```python
from build123d import *

# Parameters (mm, degrees)
ESBO_O7_R                = 1.65
RESSALTO_EXTRUS_O5_DEPTH = 8
RESSALTO_EXTRUS_O6_START = -8
ESBO_O10_R               = 1.65
RESSALTO_EXTRUS_O6_DEPTH = 8
ESBO_O8_R                = 5.5
CORTE_EXTRUS_O4_DEPTH    = 8
FILETE1_R                = 10
ESBO_O11_R               = 2.75
CORTE_EXTRUS_O5_DEPTH    = 3.5
ESBO_O14_R               = 1.75
CORTE_EXTRUS_O9_DEPTH    = 8
CORTE_EXTRUS_O10_DEPTH   = 4.9


with BuildPart() as part:
    # Esboço7 → Ressalto-extrusão5 (new body)
    with BuildSketch(Plane.XY):
        Polygon((-45.692156379, 16.70804449), (-45.692156379, -36.79195551), (6.807843621, -36.79195551), (6.807843621, 4.155908866), (3.801241904, 7.162510584), (3.84677581, 7.20804449), (3.807843621, 7.20804449), (3.807843621, 44.20804449), (-1.192156379, 49.20804449), (-23.192156379, 49.20804449), (-23.192156379, 16.70804449), align=None)
        with Locations((-1.692156379, 43.70804449)):
            Circle(ESBO_O7_R, mode=Mode.SUBTRACT)
        with Locations((-32.692156379, 0.70804449)):
            Circle(ESBO_O7_R, mode=Mode.SUBTRACT)
        with Locations((-8.692156379, 0.70804449)):
            Circle(ESBO_O7_R, mode=Mode.SUBTRACT)
    extrude(amount=RESSALTO_EXTRUS_O5_DEPTH)

    # Esboço10 → Ressalto-extrusão6 (add)
    with BuildSketch(Plane.XY.offset(8).offset(RESSALTO_EXTRUS_O6_START)):
        with BuildLine():
            Line((12.807843621, 13.70804449), (12.807843621, -31.79195551))
            ThreePointArc((12.807843621, -31.79195551), (10.464697871, -37.44880976), (4.807843621, -39.79195551))
            Line((4.807843621, -39.79195551), (-46.192156379, -39.79195551))
            ThreePointArc((-46.192156379, -39.79195551), (-51.849010628, -37.44880976), (-54.192156379, -31.79195551))
            Line((-54.192156379, -31.79195551), (-54.192156379, 13.70804449))
            ThreePointArc((-54.192156379, 13.70804449), (-50.238097925, 23.253986036), (-40.692156379, 27.20804449))
            Line((-40.692156379, 27.20804449), (-0.692156379, 27.20804449))
            ThreePointArc((-0.692156379, 27.20804449), (8.853785167, 23.253986036), (12.807843621, 13.70804449))
        make_face()
        with Locations((-8.692156379, 0.70804449)):
            Circle(ESBO_O10_R, mode=Mode.SUBTRACT)
        with Locations((-32.692156379, 0.70804449)):
            Circle(ESBO_O10_R, mode=Mode.SUBTRACT)
    extrude(amount=RESSALTO_EXTRUS_O6_DEPTH)

    # Esboço8 → Corte-extrusão4 (cut)
    with BuildSketch(Plane.XY.offset(8)):
        with Locations((-40.692156379, 13.70804449)):
            Circle(ESBO_O8_R)
        with Locations((-0.692156379, 13.70804449)):
            Circle(ESBO_O8_R)
        with Locations((-20.692156379, -26.29195551)):
            Circle(ESBO_O8_R)
    extrude(amount=-CORTE_EXTRUS_O4_DEPTH, mode=Mode.SUBTRACT)

    # Filete1
    filete1_edges = [part.edges().sort_by_distance(p)[0] for p in [
        (-23.192156379, 27.20804449, 4),
        (3.807843621, 26.435966551, 4),
    ]]
    fillet(filete1_edges, radius=FILETE1_R)

    # Esboço11 → Corte-extrusão5 (cut)
    with BuildSketch(Plane.XY.offset(8)):
        with Locations((-32.692156379, 0.70804449)):
            Circle(ESBO_O11_R)
        with Locations((-8.692156379, 0.70804449)):
            Circle(ESBO_O11_R)
        with Locations((-1.692156379, 43.70804449)):
            Circle(ESBO_O11_R)
    extrude(amount=-CORTE_EXTRUS_O5_DEPTH, mode=Mode.SUBTRACT)

    # Esboço14 → Corte-extrusão9 (cut)
    with BuildSketch(Plane.XY.offset(8)):
        with Locations((-20.692156379, 13.70804449)):
            Circle(ESBO_O14_R)
        with Locations((-40.692156379, -26.29195551)):
            Circle(ESBO_O14_R)
        with Locations((-0.692156379, -26.29195551)):
            Circle(ESBO_O14_R)
    extrude(amount=-CORTE_EXTRUS_O9_DEPTH, mode=Mode.SUBTRACT)

    # Esboço15 → Corte-extrusão10 (cut)
    with BuildSketch(Plane(origin=(0, 0, 0), x_dir=(-1, 0, 0), z_dir=(0, 0, -1))):
        Polygon((23.867582859, 13.70804449), (22.279869619, 16.45804449), (19.104443138, 16.45804449), (17.516729898, 13.70804449), (19.104443138, 10.95804449), (22.279869619, 10.95804449), align=None)
        Polygon((3.867582859, -26.29195551), (2.279869619, -23.54195551), (-0.895556862, -23.54195551), (-2.483270102, -26.29195551), (-0.895556862, -29.04195551), (2.279869619, -29.04195551), align=None)
        Polygon((43.867582859, -26.29195551), (42.279869619, -23.54195551), (39.104443138, -23.54195551), (37.516729898, -26.29195551), (39.104443138, -29.04195551), (42.279869619, -29.04195551), align=None)
    extrude(amount=-CORTE_EXTRUS_O10_DEPTH, mode=Mode.SUBTRACT)


solid = part.part
```
Could you check a few things on this model? Use its own coordinates, in mm. A direction names the side the tool comes from. Round coordinates to 2 decimals unless told otherwise and drop trailing zeros. Order: outer loops, then holes, each group sorted by start corner. A loop starts at its lowest first (then second) coordinate and runs counter-clockwise, first axis right, second up. Notation, with made-up numbers: M -14,-10.75 L 44,-10.75 A19 ccw 44,15.25 Z; hole C 58.25,49 d11. An arc over 180 degrees is marked long. One line per question, with ' | ' between items. Start each with the question number.
(1) Thinking about a two-plate mould opening in Y: for faces 1 (the face through (-3.085, -24.936, 2.416)), 2 (the face through (10.527, -37.386, 3.944)), 3 (the face through (-20, -5, 0)), which applies, +Y half, -Y half, draft (parallel to the pull), parting line (faces both ways), or undercut?
(2) Suppose I cut it at B-B on y = 10. List the corners of the cut face in (x, z) for me.
(3) For P1, Ø4, axis at y = 40.5, z = 5, coming from the +X side; P2, Ø1.5, axis at y = 31, z = 4.5, coming from the +X side; P3, Ø2, axis at x = 3.5, z = 5.5, coming from the +Y side, each with a flat end and sliding along its axis, tell me the tip position at first contact or that it passes through.
(4) Suppose I cut it at C-C on z = 6.25. Count the separate pieces of the cut face and the enclosed holes in it, then the cut area to 3 significant figures.
(5) Suppose I cut it at D-D on x = -45. List the corners of the cut face in (y, z) for me, then the cut area to 3 significant figures.
(6) Suppose I cut it at A-A on x = -32. List the corners of the cut face in (y, z) for me.
(7) Please list where these lines run through material, in increasing order: line 1 along X through (y, z) = (18, 1); line 2 along Y through (x, z) = (-43, 2.75); line 3 along X through (y, z) = (11, 7.75).
(8) For faces 4 (the face through (-23.192, 43, 4)), 5 (the face through (-18.3, 12.35, 2.42)), 6 (the face through (-54.192, -9, 4)), 7 (the face through (-8.7, -1.1, 4.5)), which set-ups out of +Z, -Z, +X, -X, +Y, -Y let a thin tool reach every point of the face, with its end or its side?
Geometry results:
1) face 1: undercut | face 2: -Y half | face 3: draft
2) outline: M -54.19,0 L -44.75,0 L -44.75,8 L -54.19,8 Z; M -36.63,0 L -4.75,0 L -4.75,8 L -36.63,8 Z; M 3.37,0 L 12.81,0 L 12.81,8 L 3.37,8 Z
3) P1: x = 3.81 | P2: x = 4 | P3: y = 45.52
4) separate pieces: 1 | enclosed holes: 9 | area: 4,610 mm²
5) outline: M -39.79,0 L 10.29,0 L 10.29,8 L -39.79,8 Z; M 17.13,0 L 26.5,0 L 26.5,8 L 17.13,8 Z | area: 476 mm²
6) outline: M -39.79,0 L -0.79,0 L -0.79,4.5 L -1.95,4.5 L -1.95,8 L -39.79,8 Z; M 2.21,0 L 27.28,0 L 27.28,8 L 3.37,8 L 3.37,4.5 L 2.21,4.5 Z
7) line 1: -53.49 to -44.13, -37.25 to -4.13, 2.75 to 12.11 | line 2: -39.79 to -27.79, -24.79 to 8.72, 18.7 to 27.01 | line 3: -54.19 to -45.48, -35.91 to -5.48, 4.09 to 12.81
8) face 4: +Z, -Z, -X, +Y | face 5: -Z | face 6: +Z, -Z, -X, +Y, -Y | face 7: +Z
